Geometry check sheet. Reference: the model listing, model coordinates, mm. A direction names the side the tool comes from. Give positions to 0.01 mm unless a question says otherwise; leave off trailing zeros. Order: outer loops, then holes, each group sorted by start corner. A loop starts at its lowest first (then second) coordinate and runs counter-clockwise, first axis right, second up.
from build123d import *

# Parameters (mm, degrees)
F0_W      = 150
F0_H      = 150
F1_DEPTH  = 75
F2_W      = 140
F2_H      = 140
F3_DEPTH  = 140
F4_R      = 4.99999
F5_W      = 70
F5_H      = 140
F6_DEPTH  = 140
F7_W      = 65
F7_H      = 140
F8_DEPTH  = 140
F9_W      = 70
F9_H      = 70
F10_DEPTH = 140
F11_W     = 70
F11_H     = 65
F12_DEPTH = 140
F13_R     = 15
F14_DEPTH = 5


# Not quite as in the source:
# - a fillet or chamfer is up to 0.001 mm smaller than in the source, because OpenCascade refuses the exact size


with BuildPart() as f1:
    # F0 (on Front) → F1 (new body, symmetric)
    with BuildSketch(Plane.XZ):
        Rectangle(F0_W, F0_H)
    extrude(amount=F1_DEPTH, both=True)

    # F2 (on face) → F3 (cut)
    with BuildSketch(Plane.XY.offset(75)):
        Rectangle(F2_W, F2_H)
    extrude(amount=-F3_DEPTH, mode=Mode.SUBTRACT)

    # F4 (radius 5 in the source; OpenCascade refuses exactly that, so slightly less here)
    f4_edges = [f1.edges().sort_by_distance(p)[0] for p in [
        (0, -75, -75),
        (75, -75, 0),
        (0, -75, 75),
        (-75, -75, 0),
        (75, 0, -75),
        (75, 75, 0),
        (75, 0, 75),
        (-75, 75, 0),
        (-75, 0, -75),
        (-75, 0, 75),
        (0, 75, -75),
        (0, 75, 75),
    ]]
    fillet(f4_edges, radius=F4_R)

    # F5 (on face) → F6 (join)
    with BuildSketch(Plane.XY.offset(-65)):
        with Locations((-35, 0)):
            Rectangle(F5_W, F5_H)
    extrude(amount=F6_DEPTH)

    # F7 (on face) → F8 (cut)
    with BuildSketch(Plane.XY.offset(75)):
        with Locations((-37.5, 0)):
            Rectangle(F7_W, F7_H)
    extrude(amount=-F8_DEPTH, mode=Mode.SUBTRACT)

    # F9 (on face) → F10 (join)
    with BuildSketch(Plane.XY.offset(-65)):
        with Locations((35, -35)):
            Rectangle(F9_W, F9_H)
    extrude(amount=F10_DEPTH)

    # F11 (on face) → F12 (cut)
    with BuildSketch(Plane.XY.offset(75)):
        with Locations((35, -37.5)):
            Rectangle(F11_W, F11_H)
    extrude(amount=-F12_DEPTH, mode=Mode.SUBTRACT)

    # F13 (on face) → F14 (join)
    with BuildSketch(Plane(origin=(0, 0, -75), x_dir=(1, 0, 0), z_dir=(0, 0, -1))):
        with Locations((-50, 50)):
            Circle(F13_R)
        with Locations((50, 50)):
            Circle(F13_R)
        with Locations((50, -50)):
            Circle(F13_R)
        with Locations((-50, -50)):
            Circle(F13_R)
    extrude(amount=F14_DEPTH)


solid = f1.part
Item 1: Set-up check for faces 5 (the flat face through (-38, 1, -65)), 6 (the cylindrical face through (38.944, -60.138, -77.465)), 7 (the cylindrical face through (1, -73, -74)): record each of +Z, -Z, +X, -X, +Y, -Y from which the full face is reachable in a straight line by a thin tool's end or side.
Reported:
face 5: +Z
face 6: -Z
face 7: -Z, +X, -X, -Y
Item 2: Scan lines: L1, parallel to Y at x = 38, z = 38.5; L2, parallel to Y at x = -65, z = -34. Record each from-to range of solid material in increasing order.
Reported:
L1: y = -75 to -70, -5 to 0, 70 to 75
L2: y = -75 to -70, 70 to 75
Item 3: Draft check along X on faces 1 (the flat face through (35, 35, -65)), 2 (the flat face through (35, -37, -65)), 3 (the cylindrical face through (-74, -1, -73)), 4 (the flat face through (-1, -75, 1)). Enter one of: released by +X, released by -X, zero draft, split by the parting line, or undercut.
Reported:
face 1: undercut
face 2: undercut
face 3: released by -X
face 4: zero draft
Item 4: Sectioned sample at C-C (z = -27.5). Enter the section's corners in (x, y), and give its area (3 significant figures).
Reported:
outline: (-75, -70) arc R5 ccw to (-70, -75) - (70, -75) arc R5 ccw to (75, -70) - (75, 70) arc R5 ccw to (70, 75) - (-70, 75) arc R5 ccw to (-75, 70) - close; hole (-70, -70) - (-5, -70) - (-5, 70) - (-70, 70) - close; hole (0, -70) - (70, -70) - (70, -5) - (0, -5) - close; hole (0, 0) - (70, 0) - (70, 70) - (0, 70) - close
area: 3,930 mm2
Item 5: Gauge pin test, flat end, axial feed: pin 1 (19.5 mm diameter, centred on x = -23.5, y = -14, fed in from +Z). Record the tip position at first contact, or that the pin passes through.
Reported:
pin 1: stops at z = -65
